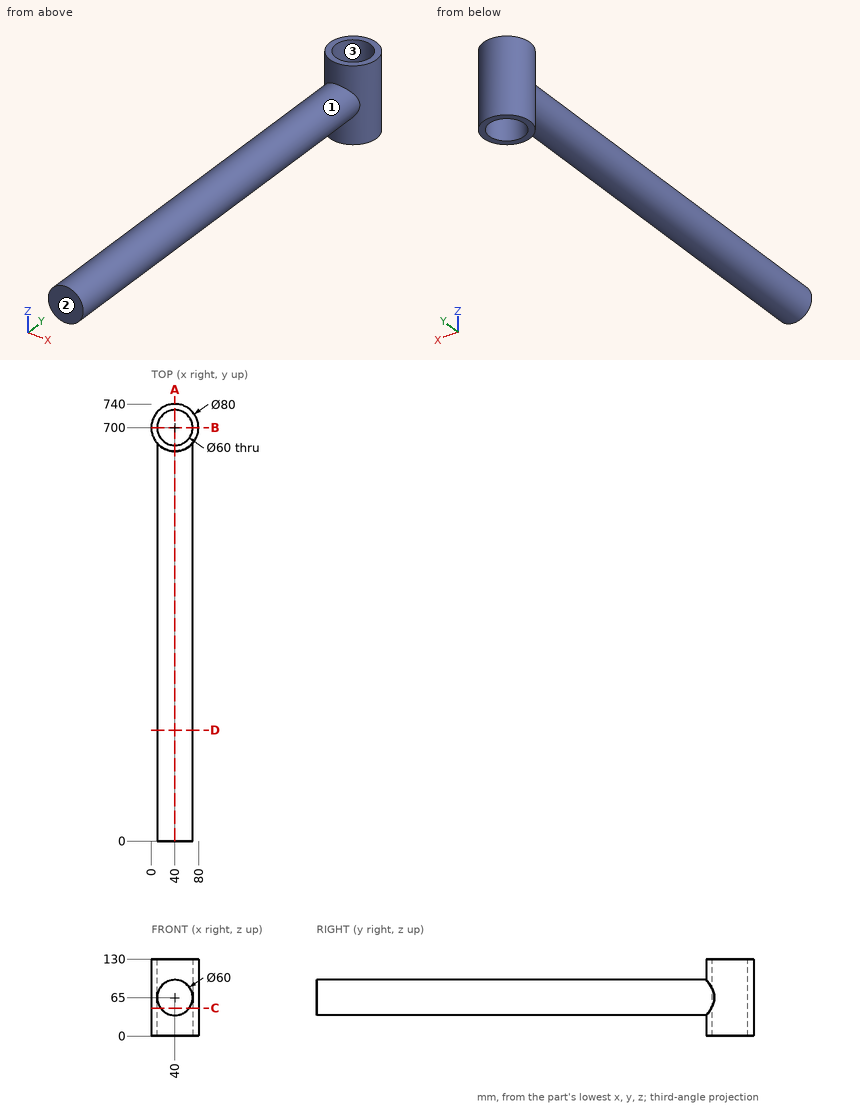
Here's the drawing with two shaded views (mm, measured from the low corner). I have some questions. Round coordinates to 2 decimals unless told otherwise and drop trailing zeros. Loops run counter-clockwise (first coordinate to the right, second up) from the corner with the lowest first, then second, coordinate; pieces in that order, holes last.
Item 1: If we mould it in two halves opening along Y, with no side actions, what happens to the marked faces 1, 2 and 3? For each: +Y half, -Y half, draft (parallel to the pull), parting line (faces both ways), or undercut.
Item 2: Suppose I cut it at A-A, the plane x = 40. Write out the boundary of the cut face in (y, z), then the cut area to 3 significant figures.
Item 3: Please list where these lines run through material, in increasing order: L1, parallel to Y at x = 39.5, z = 104; L2, parallel to Y at x = 40, z = 88.5; L3, parallel to X at y = 430.5, z = 63.5.
Item 4: Suppose I cut it at C-C, the plane z = 47. Write out the boundary of the cut face in (x, y).
Item 5: Will these pins go through, and if not, where does the flat tip stop? pin 1 Ø5 at (x, y) = (57, 492) entering from +Z; pin 2 Ø1.5 at (x, y) = (34, 482) entering from +Z; pin 3 Ø6 at (x, y) = (47.5, 164.5) entering from -Z.
Item 6: Suppose I cut it at D-D, the plane y = 188. Write out the boundary of the cut face in (x, z).
Item 7: Suppose I cut it at B-B, the plane y = 700. Write out the boundary of the cut face in (x, z).
Reported:
1. face 1: draft
1. face 2: -Y half
1. face 3: undercut
2. outline: (0, 35) - (660, 35) - (660, 0) - (670, 0) - (670, 130) - (660, 130) - (660, 95) - (0, 95) - close; (730, 0) - (740, 0) - (740, 130) - (730, 130) - close
2. area: 42,200 mm2
3. L1: y = 660 to 670, 730 to 740
3. L2: y = 0 to 670, 730 to 740
3. L3: x = 10.04 to 69.96
4. outline: (16, 0) - (64, 0) - (64, 668) arc R40 ccw (long way) to (16, 668) - close; hole circle Ø60 at (40, 700)
5. pin 1: stops at z = 91.26
5. pin 2: stops at z = 94.54
5. pin 3: stops at z = 35.34
6. outline: circle Ø60 at (40, 65)
7. outline: (0, 0) - (10, 0) - (10, 130) - (0, 130) - close; (70, 0) - (80, 0) - (80, 130) - (70, 130) - close
